from build123d import *

# Parameters (mm, degrees)
F2_DEPTH = 1
F3_DEPTH = 1
F4_R     = 1.5
F5_DEPTH = 1
F6_R     = 0.8594833568
F7_R     = 0.4


with BuildPart() as f2:
    # F0 (on Top) → F2 (new body)
    with BuildSketch(Plane.XY):
        Polygon((0, 12.0893299047), (-15, 25.9807621135), (-10.4696668122, 6.0446649524), (-30, 0), (-10.4696668122, -6.0446649524), (-15, -25.9807621135), (0, -12.0893299047), (15, -25.9807621135), (10.4696668122, -6.0446649524), (30, 0), (10.4696668122, 6.0446649524), (15, 25.9807621135), align=None)
    extrude(amount=F2_DEPTH)

    # F1 (on Top) → F3 (join)
    with BuildSketch(Plane.XY):
        with BuildLine():
            Line((72.4891722202, 37.6455299556), (7.3894136585, 5.3482959047))
            Line((7.3894136585, 5.3482959047), (7.7781090513, -6.4794942737))
            add(Edge.make_bspline(
                [(58.8173978031, 0.8565816097), (44.8322221637, -6.7676748149), (24.8244935647, -8.4759178571), (7.7781090513, -6.4794942737)],
                knots=[0, 0, 0, 0, 51.5638148865, 51.5638148865, 51.5638148865, 51.5638148865], degree=3))
            add(Edge.make_bspline(
                [(50.0547550619, 1.7504660645), (52.9756359756, 1.4525045796), (55.8965168893, 1.1545430946), (58.8173978031, 0.8565816097)],
                knots=[0, 0, 0, 0, 8.8081176893, 8.8081176893, 8.8081176893, 8.8081176893], degree=3))
            add(Edge.make_bspline(
                [(71.1085945368, 17.1669367701), (66.9464543462, 9.6644256264), (58.5000440478, 6.2858634628), (50.0547550619, 1.7504660645)],
                knots=[0, 0, 0, 0, 26.0946685292, 26.0946685292, 26.0946685292, 26.0946685292], degree=3))
            add(Edge.make_bspline(
                [(57.0727027953, 11.4145213738), (61.7513333758, 13.3319931726), (66.4299639563, 15.2494649713), (71.1085945368, 17.1669367701)],
                knots=[0, 0, 0, 0, 15.1689333795, 15.1689333795, 15.1689333795, 15.1689333795], degree=3))
            add(Edge.make_bspline(
                [(80.8876976371, 30.5125359446), (72.3214372993, 22.1036802977), (66.0250261426, 17.496548593), (57.0727027953, 11.4145213738)],
                knots=[0, 0, 0, 0, 30.5268429396, 30.5268429396, 30.5268429396, 30.5268429396], degree=3))
            add(Edge.make_bspline(
                [(57.0727027953, 19.6979995817), (65.0110344092, 23.302845036), (72.9493660231, 26.9076904903), (80.8876976371, 30.5125359446)],
                knots=[0, 0, 0, 0, 26.155461687, 26.155461687, 26.155461687, 26.155461687], degree=3))
            add(Edge.make_bspline(
                [(72.4891722202, 37.6455299556), (67.3503490786, 31.663019831), (62.2115259369, 25.6805097063), (57.0727027953, 19.6979995817)],
                knots=[0, 0, 0, 0, 23.6596994075, 23.6596994075, 23.6596994075, 23.6596994075], degree=3))
        make_face()
    extrude(amount=F3_DEPTH)

    # F4 (on face) → F5 (join)
    with BuildSketch(Plane(origin=(0, 0, 0), x_dir=(1, 0, 0), z_dir=(0, 0, -1))):
        with BuildLine():
            ThreePointArc((22.4657231152, -12.8279410816), (21.8424371227, -16.8758669464), (25.489, -15.011257492))
            ThreePointArc((25.489, -15.011257492), (25.4577954947, -14.6336770325), (25.3650286927, -14.2663419742))
            Line((25.3650286927, -14.2663419742), (22.4657231152, -12.8279410816))
        make_face()
        with Locations((23.189, -15.011257492)):
            Circle(F4_R, mode=Mode.SUBTRACT)
    extrude(amount=-F5_DEPTH)

    # F6
    f6_edges = [f2.edges().sort_by_distance(p)[0] for p in [
        (25.489, 15.011257, 0.5),
        (25.365029, 14.266342, 0.5),
        (22.465723, 12.827941, 0.5),
    ]]
    fillet(f6_edges, radius=F6_R)

    # F7
    f7_edges = [f2.edges().sort_by_distance(p)[0] for p in [
        (15, 25.980762, 0.5),
        (-15, 25.980762, 0.5),
        (-30, 0, 0.5),
        (-15, -25.980762, 0.5),
        (15, -25.980762, 0.5),
        (72.489172, 37.64553, 0.5),
        (80.887698, 30.512536, 0.5),
        (71.108595, 17.166937, 0.5),
        (58.817398, 0.856582, 0.5),
    ]]
    fillet(f7_edges, radius=F7_R)


solid = f2.part
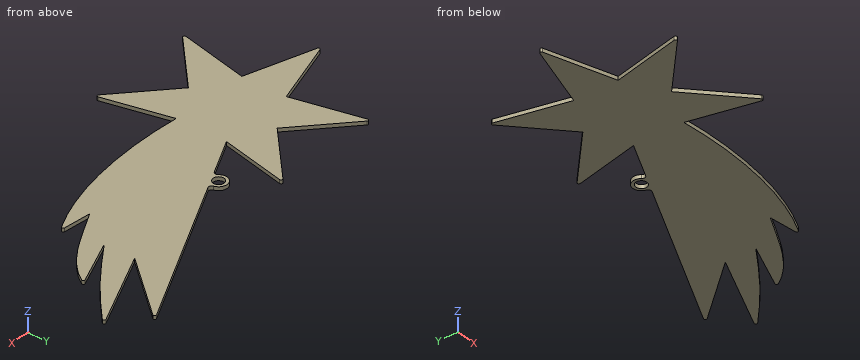
Can you work these out from the model? Positions are in its coordinate system, mm. Round coordinates to 2 decimals unless told otherwise and drop trailing zeros. Write each loop counter-clockwise with the first axis right and the second up, starting at its lowest first coordinate (ties: lowest second). Pieces come first, ordered by that corner, then holes. Notation, with made-up numbers: (23, -3) -> (36, -3) arc R18 cw to (36, 22) -> close; hole circle Ø3 at (-24.75, 21.5). An arc over 180 degrees is marked (long way). Use one line per item in the form item = value. Start each with the question number.
Q1. Imagine slicing it at B-B (x = 8.5). Please give me the cut outline in (y, z).
Q2. Imagine slicing it at A-A (x = 66). Count the separate pieces of the cut face and the enclosed holes in it, then the cut area to 3 significant figures.
Q3. If I drill on probe 1 along X at (y, z) = (19.5, 0.45); probe 2 along Y at (x, z) = (68, 0.5); probe 3 along Y at (x, z) = (23, 0.6), over which ranges is the centre line in solid material (lowest first)? Write a range as [from, to].
Q4. Imagine slicing it at C-C (x = -17). Please give me the cut outline in (y, z).
Worked out:
q1.outline = (-19.96, 0) -> (19.96, 0) -> (19.96, 1) -> (-19.96, 1) -> close
q2.separate_pieces = 3
q2.enclosed_holes = 0
q2.area = 14.3 mm^2
q3.probe_1 = [-13.53, -8], [8, 13.53], [35.91, 68.37]
q3.probe_2 = [12.98, 15.89], [19.21, 24.66], [32.42, 35.42]
q3.probe_3 = [-7.23, 13.52], [16.5, 17.3]
q4.outline = (-4.02, 0) -> (4.02, 0) -> (4.02, 1) -> (-4.02, 1) -> close
